Source: CAD feature listing. Evaluate the final solid. Frame: model axes, mm. Round coordinates to 2 decimals unless told otherwise and drop trailing zeros. Order: outer loops, then holes, each group sorted by start corner. A loop starts at its lowest first (then second) coordinate and runs counter-clockwise, first axis right, second up. Notation, with made-up numbers: (38.25, 69.5) - (76.25, 69.5) arc R9 ccw to (76.25, 77.5) - close; hole circle Ø8 at (87.25, -10.75). An arc over 180 degrees is marked (long way). Put each result on its own line as item: value. Start each with the question number.
1) Section C-C on x = -136.5. Output: boundary loops of the cut face in (y, z), then the cut area to 3 significant figures.
2) Section A-A on x = -190. Output: boundary loops of the cut face in (y, z).
3) Contact query for flat-ended pins moving along their axis: P1, Ø0.9, axis at x = -207, z = 2, coming from the -Y side; P2, Ø0.6, axis at y = 33, z = 2, coming from the -X side. Output: stop coordinate, or through.
4) Section B-B on z = 1.7. State how many separate pieces and enclosed holes the cut face has, then the cut area to 3 significant figures.
5) Line query: probe 1 along Y at (x, z) = (-364, 2.75); probe 2 along Y at (x, z) = (-315, 2.75); probe 3 along Y at (x, z) = (-210.5, 2.05). Output: solid intervals per line, ascending. Write a range as [from, to].
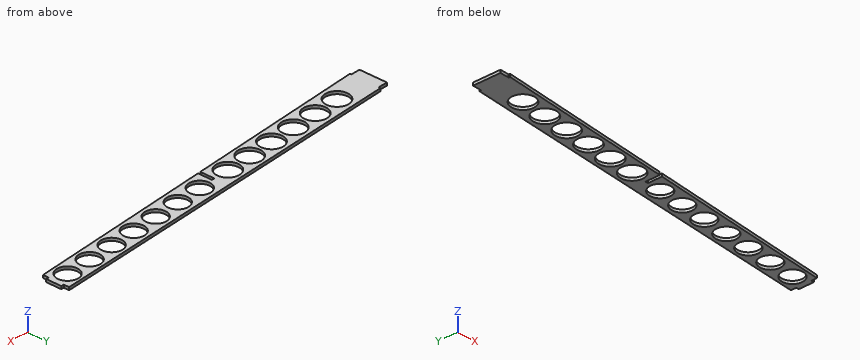
```python
from build123d import *

# Parameters (mm, degrees)
BOSS_EXTRUDE1_DEPTH     = 3
SKETCH2_R               = 12.5
SKETCH2_R_2             = 11.5
SKETCH2_W               = 3
SKETCH2_H               = 15.519078079
CUT_EXTRUDE1_DEPTH      = 1
CUT_EXTRUDE1_DEPTH_BACK = 4
SKETCH3_W               = 3
SKETCH3_H               = 6
SKETCH3_H_2             = 7.329652721
CUT_EXTRUDE2_DEPTH      = 10


with BuildPart() as part:
    # Sketch1 → Boss-Extrude1 (new body)
    with BuildSketch(Plane.XY):
        Polygon((-415, 1.5), (-415, 31.5), (-405, 31.5), (-405, 33.5), (0, 58.019626957), (0, 29.519626957), (-405, 0), (-405, 1.5), align=None)
    extrude(amount=BOSS_EXTRUDE1_DEPTH)

    # Sketch2 → Cut-Extrude1 (cut, two sides)
    with BuildSketch(Plane.XY.offset(3)) as cut_extrude1_sk:
        with Locations((-368.587798604, 18.953006079)):
            Circle(SKETCH2_R)
        with Locations((-340.175597209, 20.867070597)):
            Circle(SKETCH2_R)
        with Locations((-311.763395813, 22.781135116)):
            Circle(SKETCH2_R)
        with Locations((-283.351194418, 24.695199634)):
            Circle(SKETCH2_R)
        with Locations((-254.938993022, 26.609264153)):
            Circle(SKETCH2_R)
        with Locations((-226.526791627, 28.523328671)):
            Circle(SKETCH2_R)
        with Locations((-190, 30.98405443)):
            Circle(SKETCH2_R_2)
        with Locations((-161.331258472, 32.915401465)):
            Circle(SKETCH2_R_2)
        with Locations((-132.662516945, 34.846748501)):
            Circle(SKETCH2_R_2)
        with Locations((-103.993775417, 36.778095537)):
            Circle(SKETCH2_R_2)
        with Locations((-75.325033889, 38.709442573)):
            Circle(SKETCH2_R_2)
        with Locations((-46.656292362, 40.640789609)):
            Circle(SKETCH2_R_2)
        with Locations((-17.987550834, 42.572136645)):
            Circle(SKETCH2_R_2)
        with Locations((-207.5, 22.045580728)):
            Rectangle(SKETCH2_W, SKETCH2_H)
    extrude(amount=CUT_EXTRUDE1_DEPTH, mode=Mode.SUBTRACT)
    extrude(cut_extrude1_sk.sketch, amount=-CUT_EXTRUDE1_DEPTH_BACK, mode=Mode.SUBTRACT)

    # Sketch3 → Cut-Extrude2 (cut)
    with BuildSketch(Plane.XY.offset(3)):
        with Locations((-1.5, 55.019626957)):
            Rectangle(SKETCH3_W, SKETCH3_H)
        with Locations((-1.5, 31.854800596)):
            Rectangle(SKETCH3_W, SKETCH3_H_2)
    extrude(amount=-CUT_EXTRUDE2_DEPTH, mode=Mode.SUBTRACT)


solid = part.part
```
Answer sheet:
1. outline: (19.57, 0) - (24.01, 0) - (24.01, 3) - (19.57, 3) - close; (45.69, 0) - (49.76, 0) - (49.76, 3) - (45.69, 3) - close
1. area: 25.5 mm^2
2. outline: (15.67, 0) - (19.48, 0) - (19.48, 3) - (15.67, 3) - close; (42.48, 0) - (46.52, 0) - (46.52, 3) - (42.48, 3) - close
3. P1: y = 29.81
3. P2: x = -405
4. separate pieces: 1
4. enclosed holes: 13
4. area: 6,920 mm^2
5. probe 1: [2.99, 7.33], [30.58, 35.98]
5. probe 2: [6.56, 10.71], [34.85, 38.95]
5. probe 3: [14.18, 45.28]
